```python
from build123d import *

# Parameters (mm, degrees)
F0_W     = 63.5
F0_H     = 6.35
F1_DEPTH = 190.5
F3_DEPTH = 25.4
F5_DEPTH = 25.4
F7_DEPTH = 3.175


with BuildPart() as f1:
    # F0 (on Top) → F1 (new body)
    with BuildSketch(Plane.XY):
        with BuildLine():
            Line((51.371804, 0), (-12.128196, 0))
            ThreePointArc((-12.128196, 0), (19.621804, -16.493909), (51.371804, 0))
        make_face()
        with Locations((19.621804, 3.175)):
            Rectangle(F0_W, F0_H)
    extrude(amount=F1_DEPTH)

    # F2 (on face) → F3 (cut)
    with BuildSketch(Plane(origin=(0, 6.35, 0), x_dir=(-1, 0, 0), z_dir=(0, 1, 0))):
        Polygon((-51.371804, 190.5), (-51.371804, 0), (-46.952475, 190.5), align=None)
        Polygon((8.916664, 190.5), (12.128196, 0), (12.128196, 190.5), align=None)
    extrude(amount=-F3_DEPTH, mode=Mode.SUBTRACT)

    # F4 (on face) → F5 (cut)
    with BuildSketch(Plane(origin=(0, 6.35, 0), x_dir=(-1, 0, 0), z_dir=(0, 1, 0))):
        with BuildLine():
            Line((-51.371804, 0), (12.128196, 0))
            ThreePointArc((12.128196, 0), (-19.621804, 7.10176), (-51.371804, 0))
        make_face()
    extrude(amount=-F5_DEPTH, mode=Mode.SUBTRACT)

    # F6 (on face) → F7 (join)
    with BuildSketch(Plane(origin=(0, 6.35, 0), x_dir=(-1, 0, 0), z_dir=(0, 1, 0))):
        Polygon((8.916664, 190.5), (-46.952475, 190.5), (-47.011383, 187.960683), (8.959473, 187.960683), align=None)
    extrude(amount=F7_DEPTH)


solid = f1.part
```
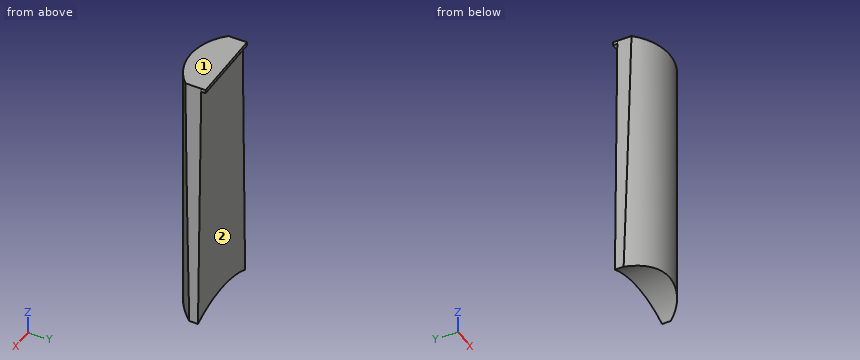
Input: part model. Units: mm. Frame: model coordinates. Face numbers are marked on the shaded views. A direction names the side the tool comes from. Give positions to 0.01 mm unless a question says otherwise; leave off trailing zeros. Order: outer loops, then holes, each group sorted by start corner. A loop starts at its lowest first (then second) coordinate and runs counter-clockwise, first axis right, second up.
1. Section A-A on x = 15. Return the cut outline in (y, z) (3 decimals), and give its area (3 significant figures).
Derived:
outline: (-16.218, 6.958) - (6.35, 6.958) - (6.35, 187.961) - (9.525, 187.961) - (9.525, 190.5) - (-16.218, 190.5) - close
area: 4,150 mm2
2. Pin query (flat end, axial travel): pin 1 (3.5 mm diameter, centred on x = 26.5, y = 7.5, fed in from -Z); pin 2 (2 mm diameter, centred on y = 4.5, z = 83.5, fed in from +X); pin 3 (8 mm diameter, centred on y = 1, z = 60.5, fed in from -X); pin 4 (1 mm diameter, centred on x = -1, y = -12.5, fed in from +Z). Return the tip coordinate at first contact, or that it passes through.
Derived:
pin 1: stops at z = 6.65
pin 2: stops at x = 49.46
pin 3: stops at x = -11.18
pin 4: passes through
3. Section C-C on z = 107. Return the cut outline in (x, y), and give its area (3 significant figures).
Derived:
outline: (-10.32, -2.37) arc R38.81 ccw to (48.89, -3.17) - (48.89, 6.35) - (-10.32, 6.35) - close
area: 1,100 mm2
4. Section B-B on y = 4. Return the cut outline in (x, z), and give its area (3 significant figures).
Derived:
outline: (-12.13, 0) arc R74.52 cw to (51.37, 0) - (46.95, 190.5) - (-8.92, 190.5) - close
area: 11,100 mm2
5. Material intervals for L1, parallel to Z at x = 20, y = 2.25; L2, parallel to X at y = -8.5, z = 41; L3, parallel to Y at x = 38.5, z = 106, sorted ascending.
Derived:
L1: z = 7.1 to 190.5
L2: x = -3.97 to 43.21
L3: y = -11.59 to 6.35
6. Reachability of the marked faces 1 and 2 from +Z, -Z, +X, -X, +Y, -Y: full face, straight path, thin tool, end or side. Return the list, or none.
Derived:
face 1: +Z, +X, -X, +Y, -Y
face 2: -Z, +X, -X, +Y
7. Section D-D on x = -0.5. Return the cut outline in (y, z) (3 decimals), and give its area (3 significant figures).
Derived:
outline: (-10.869, 4.334) - (6.35, 4.334) - (6.35, 187.961) - (9.525, 187.961) - (9.525, 190.5) - (-10.869, 190.5) - close
area: 3,210 mm2
